```python
from build123d import *

# Parameters (mm, degrees)
BASE_EXTRUDE_THIN_DEPTH = 76
BOSS_EXTRUDE1_START     = -8
BOSS_EXTRUDE1_DEPTH     = 8
SKETCH3_W               = 87.757240917
SKETCH3_H               = 51
BOSS_EXTRUDE2_DEPTH     = 8
CUT_EXTRUDE1_DEPTH      = 119.888876867
FILLET1_R               = 12.5
BOSS_EXTRUDE3_DEPTH     = 10
CUT_EXTRUDE2_DEPTH      = 101.073742043
SKETCH9_R               = 8
CUT_EXTRUDE3_DEPTH      = 118.428403891
LPATTERN2_COUNT         = 2
LPATTERN2_PITCH         = 28


# Read off the part's stored shape, not the designer's step: Boss-Extrude1
with BuildPart() as part:
    # Sketch1 → Base-Extrude-Thin (new body)
    with BuildSketch(Plane(origin=(0, 0, 0), x_dir=(0, 0, -1), z_dir=(1, 0, 0))):
        Polygon((-38, 0), (0, 0), (0, 32), (8, 32), (8, -8), (-38, -8), align=None)
    extrude(amount=BASE_EXTRUDE_THIN_DEPTH)

    # Boss-Extrude1 outline → Boss-Extrude1 (add)
    with BuildSketch(Plane.XY.offset(BOSS_EXTRUDE1_START)):
        Polygon((76, 32), (0, 75.878620458), (0, 32), align=None)
    extrude(amount=BOSS_EXTRUDE1_DEPTH)

    # Sketch3 → Boss-Extrude2 (add)
    with BuildSketch(Plane(origin=(32.856406461, 56.908965344, 0), x_dir=(-0.8660254037844379, 0.5000000000000014, 0), z_dir=(0.5000000000000014, 0.8660254037844379, 0))):
        with Locations((-5.93931023, -25.5)):
            Rectangle(SKETCH3_W, SKETCH3_H)
    extrude(amount=-BOSS_EXTRUDE2_DEPTH)

    # Sketch4 → Cut-Extrude1 (cut, through all)
    with BuildSketch(Plane.XY):
        Polygon((-113.800448301, -130.46714223), (0, 66.641016151), (4, 73.569219382), (117.800448301, 270.677377763), (-276.415868462, 498.278274366), (-508.016765065, 97.133754372), align=None)
    extrude(amount=-CUT_EXTRUDE1_DEPTH, mode=Mode.SUBTRACT)

    # Fillet1
    fillet1_edges = [part.edges().sort_by_distance(p)[0] for p in [
        (74, 28.535898385, -51),
        (2, 70.105117767, -51),
    ]]
    fillet(fillet1_edges, radius=FILLET1_R)

    # Sketch5 → Boss-Extrude3 (add)
    with BuildSketch(Plane.ZY):
        Polygon((0, 38), (0, 0), (38, 0), align=None)
    extrude(amount=-BOSS_EXTRUDE3_DEPTH)

    # Sketch6 → Cut-Extrude2 (cut, through all)
    with BuildSketch(Plane(origin=(24.713169413, 61.610465445, -0.61351416), x_dir=(-0.866025403784438, 0.5000000000000012, 0), z_dir=(0.5000000000000011, 0.8660254037844379, 0))):
        with BuildLine():
            Line((-1.220930891, -34.88648584), (-22.388771324, -34.88648584))
            ThreePointArc((-22.388771324, -34.88648584), (-47.720930891, -28.38648584), (-22.388771324, -21.88648584))
            Line((-22.388771324, -21.88648584), (-1.220930891, -21.88648584))
            ThreePointArc((-1.220930891, -21.88648584), (5.279069109, -28.38648584), (-1.220930891, -34.88648584))
        make_face()
    extrude(amount=-CUT_EXTRUDE2_DEPTH, mode=Mode.SUBTRACT)

    # Sketch9 → Cut-Extrude3 (cut, through all)
    with BuildSketch(Plane(origin=(0, 0, 0), x_dir=(-1, 0, 0), z_dir=(0, 1, 0))):
        with Locations(Location((-60, 19, 0), (0, 0, 90))):
            Circle(SKETCH9_R)
    cut_extrude3 = extrude(amount=-CUT_EXTRUDE3_DEPTH, mode=Mode.SUBTRACT)

    # LPattern2: Cut-Extrude3 ×2
    with Locations(*[(-i * LPATTERN2_PITCH, 0, 0) for i in range(1, LPATTERN2_COUNT)]):
        add(cut_extrude3, mode=Mode.SUBTRACT)


solid = part.part
```
Here's how the part is built. I have some questions about the finished solid (model axes, mm). A direction names the side the tool comes from. Coordinates: 2 decimals unless noted, no trailing zeros. Loops run counter-clockwise (first coordinate to the right, second up) from the corner with the lowest first, then second, coordinate; pieces in that order, holes last. Notation, with made-up numbers: M 18.25,-17 L 73.25,-17 A21 ccw 73.25,10 Z; hole C -39.5,5.5 d1. An arc over 180 degrees is marked long. One line per item, written item: value.
1. Please list where these lines run through material, in increasing order: probe 1 along X at (y, z) = (-6, 19); probe 2 along Z at (x, y) = (29.5, 56.5); probe 3 along Z at (x, y) = (29.5, 16).
Geometry says:
probe 1: x = 0 to 24, 40 to 52, 68 to 76
probe 2: z = -51 to -35.5, -22.5 to 0
probe 3: z = -8 to 0
2. Imagine slicing it at B-B (z = -19). List the corners of the cut face in (x, y) for me.
Geometry says:
outline: M 0,66.64 L 42.5,42.11 L 46.5,49.03 L 4,73.57 Z; M 58.2,33.04 L 72,25.07 L 76,32 L 62.2,39.97 Z
3. Imagine slicing it at C-C (y = 18). List the corners of the cut face in (x, z) for me, and give its area (3 significant figures).
Geometry says:
outline: M 0,-8 L 76,-8 L 76,0 L 10,0 L 10,20 L 0,20 Z
area: 808 mm2
4. Imagine slicing it at D-D (x = 32). List the corners of the cut face in (y, z) for me, and give its area (3 significant figures).
Geometry says:
outline: M -8,-8 L 48.17,-8 L 48.17,-22.5 L 57.4,-22.5 L 57.4,0 L 0,0 L 0,11 L -8,11 Z; M -8,27 L 0,27 L 0,38 L -8,38 Z; M 48.17,-51 L 57.4,-51 L 57.4,-35.5 L 48.17,-35.5 Z
area: 976 mm2
5. Thinking about a two-plate mould opening in X: for faces 1 (the cylindrical face through (18.17, 60.83, -28.86)), 2 (the cylindrical face through (39.932, -3.944, 17.959)), 3 (the flat face through (43, 0, 19)), which applies, +X half, -X half, draft (parallel to the pull), parting line (faces both ways), or undercut?
Geometry says:
face 1: +X half
face 2: undercut
face 3: draft
6. Will these pins go through, and if not, where does the flat tip stop? pin 1 Ø1.5 at (x, z) = (46.5, -18.5) entering from +Y; pin 2 Ø9.5 at (x, z) = (60, 19) entering from -Y; pin 3 Ø5 at (y, z) = (26, -22) entering from +X; pin 4 Ø4 at (x, z) = (56, 26.5) entering from +Y.
Geometry says:
pin 1: stops at y = 49.46
pin 2: passes through
pin 3: stops at x = 73.98
pin 4: stops at y = 0
7. On a 3-axis mill with a long thin cutter (end or side, diameter ignored), from which of +Z, -Z, +X, -X, +Y, -Y can I reach the whole of each face in a straight line? I mean faces 4 (the flat face through (36.5, 45.57, -19.64)), 5 (the flat face through (36, 28, 0)), 6 (the flat face through (0, 22, 4)), 7 (the flat face through (74.028, 28.584, -23.463)). Say none if no direction works.
Geometry says:
face 4: -Z, -X, -Y
face 5: +Z, +X, +Y
face 6: +Z, -Z, -X, +Y, -Y
face 7: -Z, +X, -Y
8. Imagine slicing it at A-A (z = 19). List the corners of the cut face in (x, y) for me.
Geometry says:
outline: M 0,-8 L 24,-8 L 24,0 L 10,0 L 10,19 L 0,19 Z; M 40,-8 L 52,-8 L 52,0 L 40,0 Z; M 68,-8 L 76,-8 L 76,0 L 68,0 Z
